Check sheet for the modelled part. Datum: model origin and axes. Units: mm. Face numbers are marked on the shaded views. A direction names the side the tool comes from. Round coordinates to 2 decimals unless told otherwise and drop trailing zeros. Write each loop counter-clockwise with the first axis right and the second up, starting at its lowest first coordinate (ties: lowest second). Pieces come first, ordered by that corner, then holes. Notation, with made-up numbers: (19.25, -36.5) -> (53.25, -36.5) arc R23 cw to (53.25, -24.5) -> close; hole circle Ø3 at (20.5, -2.75). An arc over 180 degrees is marked (long way). Put each result on its own line as item: value. Start each with the question number.
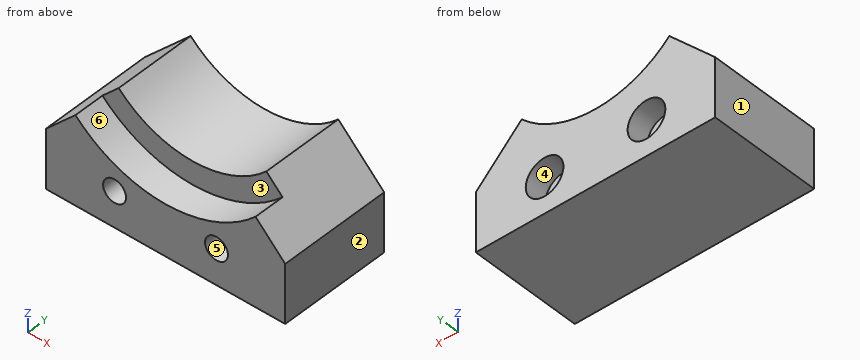
from build123d import *

# Parameters (mm, degrees)
PAD046_DEPTH     = 22
SKETCH_R         = 25
POCKET_DEPTH     = 6
HOLE_D           = 4.5
HOLE_CBORE_D     = 7.4
HOLE_CBORE_DEPTH = 4.4


with BuildPart() as part:
    # Sketch078 → Pad046 (new body)
    with BuildSketch(Plane.XZ.offset(-27)):
        with BuildLine():
            Line((-23.5, -35), (23.5, -35))
            Line((23.5, -35), (23.5, -23.5))
            Line((14.495689, -14.495689), (23.5, -23.5))
            ThreePointArc((-14.495689, -14.495689), (0, -20.5), (14.495689, -14.495689))
            Line((-23.5, -23.5), (-14.495689, -14.495689))
            Line((-23.5, -23.5), (-23.5, -35))
        make_face()
    extrude(amount=-PAD046_DEPTH)

    # Sketch → Pocket (cut)
    with BuildSketch(Plane.XZ.offset(-27)):
        Circle(SKETCH_R)
    extrude(amount=-POCKET_DEPTH, mode=Mode.SUBTRACT)

    # Hole (through all)
    with Locations(Plane(origin=(0, 49, 0), x_dir=(1, 0, 0), z_dir=(0, 1, 0))):
        with Locations((-10, 28), (10, 28)):
            CounterBoreHole(HOLE_D / 2, HOLE_CBORE_D / 2, HOLE_CBORE_DEPTH)


solid = part.part
1. Access from +Z, -Z, +X, -X, +Y, -Y to the whole of each face (thin tool, end or side, straight path). Record for the marked faces 4, 5 and 6.
2. Section check C-C, the plane x = -10. Enter the section's corners in (y, z).
3. Gauge pin test, flat ends, axial feed: P1, Ø12, axis at x = 1.5, y = 36.5, coming from the +Z side; P2, Ø8.5, axis at x = 3.5, z = -18, coming from the -Y side; P3, Ø4, axis at x = -18.5, y = 34, coming from the +Z side; P4, Ø3.5, axis at x = 10, z = -28, coming from the -Y side. Record the tip position at first contact, or that the pin passes through.
4. Draft check along X on the marked faces 1, 2 and 3. Enter one of: released by +X, released by -X, zero draft, split by the parting line, or undercut.
5. Section check D-D, the plane z = -28. Enter the section's corners in (x, y).
6. Section check B-B, the plane y = 46. Enter the section's corners in (x, z).
7. Material ranges on L1, parallel to X at y = 36.75, z = -28; L2, parallel to X at y = 47, z = -28; L3, parallel to X at y = 40.25, z = -18.75, recorded low to high. Write a range as [from, to].
8. Section check A-A, the plane z = -20. Enter the section's corners in (x, y), then the cut area to 3 significant figures.
Reply:
1. face 4: +Y
1. face 5: +Y, -Y
1. face 6: +Z, -Y
2. outline: (27, -35) -> (49, -35) -> (49, -31.7) -> (44.6, -31.7) -> (44.6, -30.25) -> (27, -30.25) -> close; (27, -25.75) -> (44.6, -25.75) -> (44.6, -24.3) -> (49, -24.3) -> (49, -17.9) -> (33, -17.9) -> (33, -22.91) -> (27, -22.91) -> close
3. P1: stops at z = -19.08
3. P2: stops at y = 33
3. P3: stops at z = -16.5
3. P4: passes through
4. face 1: released by -X
4. face 2: released by +X
4. face 3: undercut
5. outline: (-23.5, 27) -> (-12.25, 27) -> (-12.25, 44.6) -> (-13.7, 44.6) -> (-13.7, 49) -> (-23.5, 49) -> close; (-7.75, 27) -> (7.75, 27) -> (7.75, 44.6) -> (6.3, 44.6) -> (6.3, 49) -> (-6.3, 49) -> (-6.3, 44.6) -> (-7.75, 44.6) -> close; (12.25, 27) -> (23.5, 27) -> (23.5, 49) -> (13.7, 49) -> (13.7, 44.6) -> (12.25, 44.6) -> close
6. outline: (-23.5, -35) -> (23.5, -35) -> (23.5, -23.5) -> (14.5, -14.5) arc R20.5 cw to (-14.5, -14.5) -> (-23.5, -23.5) -> close; hole circle Ø7.4 at (-10, -28); hole circle Ø7.4 at (10, -28)
7. L1: x = [-23.5, -12.25], [-7.75, 7.75], [12.25, 23.5]
7. L2: x = [-23.5, -13.7], [-6.3, 6.3], [13.7, 23.5]
7. L3: x = [-18.75, -8.29], [8.29, 18.75]
8. outline: (-20, 27) -> (-15, 27) -> (-15, 33) -> (-4.5, 33) -> (-4.5, 49) -> (-20, 49) -> close; (4.5, 33) -> (15, 33) -> (15, 27) -> (20, 27) -> (20, 49) -> (4.5, 49) -> close
8. area: 556 mm2
